Part model, mm, in its own coordinate system. A direction names the side the tool comes from. Round coordinates to 2 decimals unless told otherwise and drop trailing zeros. Write each loop counter-clockwise with the first axis right and the second up, starting at its lowest first coordinate (ties: lowest second). Pieces come first, ordered by that corner, then holes. Notation, with made-up numbers: (-38.5, 42.5) -> (-13.5, 42.5) arc R17 cw to (-13.5, 56.5) -> close; hole circle Ø7 at (-27, 34). An arc over 180 degrees is marked (long way). Return JSON: item names as keys, results as strings. Group by question number.
(1) Saw through at B-B (y = 6.25). List the corners of the cut face in (x, z).
(2) Drill centre lines: L1, parallel to Z at x = 37, y = 6; L2, parallel to X at y = 7, z = -40; L3, parallel to Z at x = 21, y = 5.25. Where is each one in solid material? Low to high. Write a range as from..to.
(3) Tool access for faces 1 (the flat face through (-1, 1, -15)), 2 (the flat face through (25.351, 5.944, -33.936)), 3 (the cylindrical face through (37.37, 5.94, -38.34)): list every direction of +Z, -Z, +X, -X, +Y, -Y with a clear straight run to the whole face (end or side of a thin tool).
(4) Saw through at A-A (x = 37). List the corners of the cut face in (y, z), plus the area to 3 significant figures.
(5) Saw through at D-D (x = 19). List the corners of the cut face in (y, z).
(6) Drop flat-ended pins along their axis: pin 1 Ø2 at (x, y) = (8, 7.5) entering from -Z; pin 2 Ø2.5 at (x, z) = (37, -40) entering from -Y; pin 3 Ø2 at (x, y) = (-20.5, 1.5) entering from -Z; pin 4 Ø5 at (x, z) = (-34.5, -32.5) entering from -Y. Give the stop position or say it passes through.
(7) Saw through at C-C (z = -30.5). List the corners of the cut face in (x, y).
(8) Mould opens along X. For faces 4 (the flat face through (45, 5, -20)), 5 (the flat face through (-45, 5, -20)), 6 (the flat face through (1, 5, 0)), 7 (the flat face through (0, 6, -25)) say: +X half, -X half, draft (parallel to the pull), parting line (faces both ways), or undercut.
from build123d import *

# Parameters (mm, degrees)
BOSS_EXTRUDE1_DEPTH      = 10
SKETCH2_W                = 85
SKETCH2_H                = 33
CUT_EXTRUDE1_DEPTH       = 2
FILLET1_R                = 1
M3_CLEARANCE_HOLE1_D     = 3.4
M3_CLEARANCE_HOLE1_DEPTH = 8
M3_CLEARANCE_HOLE1_TIP   = 1.021463052


with BuildPart() as part:
    # Sketch1 → Boss-Extrude1 (new body)
    with BuildSketch(Plane(origin=(0, 0, 0), x_dir=(1, 0, 0), z_dir=(0, 1, 0))):
        with BuildLine():
            Line((45, 0), (-45, 0))
            Line((-45, 0), (-45, 40))
            ThreePointArc((-45, 40), (-38.595106732, 47.83936442), (-29.636091372, 43.126155741))
            Line((-29.636091372, 43.126155741), (-21.183726137, 25))
            Line((-21.183726137, 25), (21.183726137, 25))
            Line((21.183726137, 25), (29.636091372, 43.126155741))
            ThreePointArc((29.636091372, 43.126155741), (38.595106732, 47.83936442), (45, 40))
            Line((45, 40), (45, 0))
        make_face()
    extrude(amount=BOSS_EXTRUDE1_DEPTH)

    # Sketch2 → Cut-Extrude1 (cut)
    with BuildSketch(Plane.XZ):
        with Locations((0, -31.5)):
            Rectangle(SKETCH2_W, SKETCH2_H)
    extrude(amount=-CUT_EXTRUDE1_DEPTH, mode=Mode.SUBTRACT)

    # Fillet1
    fillet1_edges = [part.edges().sort_by_distance(p)[0] for p in [
        (42.5, 1, -15),
        (-42.5, 1, -15),
    ]]
    fillet(fillet1_edges, radius=FILLET1_R)

    # M3 Clearance Hole1
    with Locations(Plane(origin=(0, 10, 0), x_dir=(1, 0, 0), z_dir=(0, 1, 0))):
        with Locations((-37, 40), (37, 40)):
            Hole(M3_CLEARANCE_HOLE1_D / 2, depth=M3_CLEARANCE_HOLE1_DEPTH)
            with Locations((0, 0, -(M3_CLEARANCE_HOLE1_DEPTH + M3_CLEARANCE_HOLE1_TIP / 2))):  # 118° drill point
                Cone(0, M3_CLEARANCE_HOLE1_D / 2, M3_CLEARANCE_HOLE1_TIP, mode=Mode.SUBTRACT)


solid = part.part
Computed values:
{
 "1": {"outline": "(-45, -40) arc R8 ccw to (-29.64, -43.13) -> (-21.18, -25) -> (21.18, -25) -> (29.64, -43.13) arc R8 ccw to (45, -40) -> (45, 0) -> (-45, 0) -> close; hole circle Ø3.4 at (-37, -40); hole circle Ø3.4 at (37, -40)"},
 "2": {"L1": "-48..-41.7, -38.3..0", "L2": "-45..-38.7, -35.3..-28.18, 28.18..35.3, 38.7..45", "L3": "-25..0"},
 "3": {"face 1": "-Z, -Y", "face 2": "-Z, +Y, -Y", "face 3": "+Y, -Y"},
 "4": {"outline": "(0, -15) -> (2, -15) -> (2, -38.3) -> (10, -38.3) -> (10, 0) -> (0, 0) -> close; (2, -48) -> (10, -48) -> (10, -41.7) -> (2, -41.7) -> close", "area": "387 mm2"},
 "5": {"outline": "(0, -15) -> (2, -15) -> (2, -25) -> (10, -25) -> (10, 0) -> (0, 0) -> close"},
 "6": {"pin 1": "z = -25", "pin 2": "through", "pin 3": "z = -25.39", "pin 4": "y = 2"},
 "7": {"outline": "(-45, 0) -> (-42.5, 0) -> (-42.5, 2) -> (-23.75, 2) -> (-23.75, 10) -> (-45, 10) -> close; (23.75, 2) -> (42.5, 2) -> (42.5, 0) -> (45, 0) -> (45, 10) -> (23.75, 10) -> close"},
 "8": {"face 4": "+X half", "face 5": "-X half", "face 6": "draft", "face 7": "undercut"}
}
